```python
from build123d import *

# Parameters (mm, degrees)
SKETCH1_R           = 17.8689
BOSS_EXTRUDE1_DEPTH = 2.921
SKETCH2_R           = 10.795
BOSS_EXTRUDE2_DEPTH = 9.398
CUT_EXTRUDE1_DEPTH  = 29.113216383
SKETCH4_R           = 2.413
CUT_EXTRUDE2_DEPTH  = 16.002


with BuildPart() as part:
    # Sketch1 → Boss-Extrude1 (new body)
    with BuildSketch(Plane.XY):
        Circle(SKETCH1_R)
    extrude(amount=BOSS_EXTRUDE1_DEPTH)

    # Sketch2 → Boss-Extrude2 (add)
    with BuildSketch(Plane.XY.offset(2.921)):
        Circle(SKETCH2_R)
    extrude(amount=BOSS_EXTRUDE2_DEPTH)

    # Sketch3 → Cut-Extrude1 (cut, through all)
    with BuildSketch(Plane.XY.offset(12.319)):
        with BuildLine():
            Line((-3.77825, -3.274862888), (-3.77825, 3.274862888))
            ThreePointArc((-3.77825, 3.274862888), (0, 4.99999), (3.77825, 3.274862888))
            Line((3.77825, 3.274862888), (3.77825, -3.274862888))
            ThreePointArc((3.77825, -3.274862888), (0, -4.99999), (-3.77825, -3.274862888))
        make_face()
    extrude(amount=-CUT_EXTRUDE1_DEPTH, mode=Mode.SUBTRACT)

    # Sketch4 → Cut-Extrude2 (cut)
    with BuildSketch(Plane(origin=(0, 0, 0), x_dir=(0, 0, -1), z_dir=(1, 0, 0))):
        with Locations(Location((-7.6962, 0, 0), (0, 0, 180))):
            Circle(SKETCH4_R)
    extrude(amount=-CUT_EXTRUDE2_DEPTH, mode=Mode.SUBTRACT)


solid = part.part
```
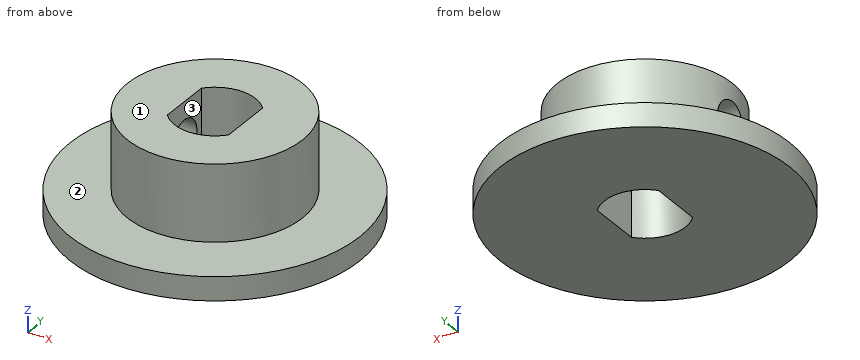
Input: part model. Units: mm. Frame: model coordinates. Face numbers are marked on the shaded views. A direction names the side the tool comes from. Coordinates: 2 decimals unless noted, no trailing zeros. Loops run counter-clockwise (first coordinate to the right, second up) from the corner with the lowest first, then second, coordinate; pieces in that order, holes last.
Q1. Section B-B, the plane x = 0. Return the cut outline in (y, z) (3 decimals).
Results are:
outline: (-17.869, 0) - (-5, 0) - (-5, 12.319) - (-10.795, 12.319) - (-10.795, 2.921) - (-17.869, 2.921) - close; (5, 0) - (17.869, 0) - (17.869, 2.921) - (10.795, 2.921) - (10.795, 12.319) - (5, 12.319) - close
Q2. Section C-C, the plane z = 11.5. Return the cut outline in (x, y) (3 decimals).
Results are:
outline: circle Ø21.59 at (0, 0); hole (-3.778, -3.275) arc R5 ccw to (3.778, -3.275) - (3.778, 3.275) arc R5 ccw to (-3.778, 3.275) - close
Q3. Section A-A, the plane y = 0. Return the cut outline in (x, z) (3 decimals).
Results are:
outline: (-17.869, 0) - (-3.778, 0) - (-3.778, 5.283) - (-10.795, 5.283) - (-10.795, 2.921) - (-17.869, 2.921) - close; (-10.795, 10.109) - (-3.778, 10.109) - (-3.778, 12.319) - (-10.795, 12.319) - close; (3.778, 0) - (17.869, 0) - (17.869, 2.921) - (10.795, 2.921) - (10.795, 12.319) - (3.778, 12.319) - close
Q4. Section D-D, the plane z = 8.5. Return the cut outline in (x, y) (3 decimals).
Results are:
outline: (-10.553, -2.275) arc R10.795 ccw (long way) to (-10.553, 2.275) - (-3.778, 2.275) - (-3.778, 3.275) arc R5 cw to (3.778, 3.275) - (3.778, -3.275) arc R5 cw to (-3.778, -3.275) - (-3.778, -2.275) - close
Q5. Set-up query: the marked faces 1, 2 and 3. Return all of +Z, -Z, +X, -X, +Y, -Y with unobstructed straight access to the full face (end or side cutting, diameter ignored); none if empty.
Results are:
face 1: +Z, +X, -X, +Y, -Y
face 2: +Z
face 3: +Z, -Z
Q6. Line query: line 1 along Z through (x, y) = (6, -12.5); line 2 along Y through (x, z) = (-7.5, 7.5); line 3 along Y through (x, z) = (-0.5, 6.5). Output: solid intervals per line, ascending.
Results are:
line 1: z = 0 to 2.92
line 2: y = -7.76 to -2.41, 2.41 to 7.76
line 3: y = -10.78 to -4.97, 4.97 to 10.78
Q7. Contact query for flat-ended pins moving along their axis: pin 1 (2 mm diameter, centred on x = 6, y = 11.5, fed in from +Z); pin 2 (5 mm diameter, centred on y = 1, z = 6.5, fed in from -X) (3 decimals); pin 3 (4 mm diameter, centred on x = 10, z = 6, fed in from -Y). Output: stop coordinate, or through.
Results are:
pin 1: stops at z = 2.92
pin 2: stops at x = -10.795
pin 3: stops at y = -7.25
